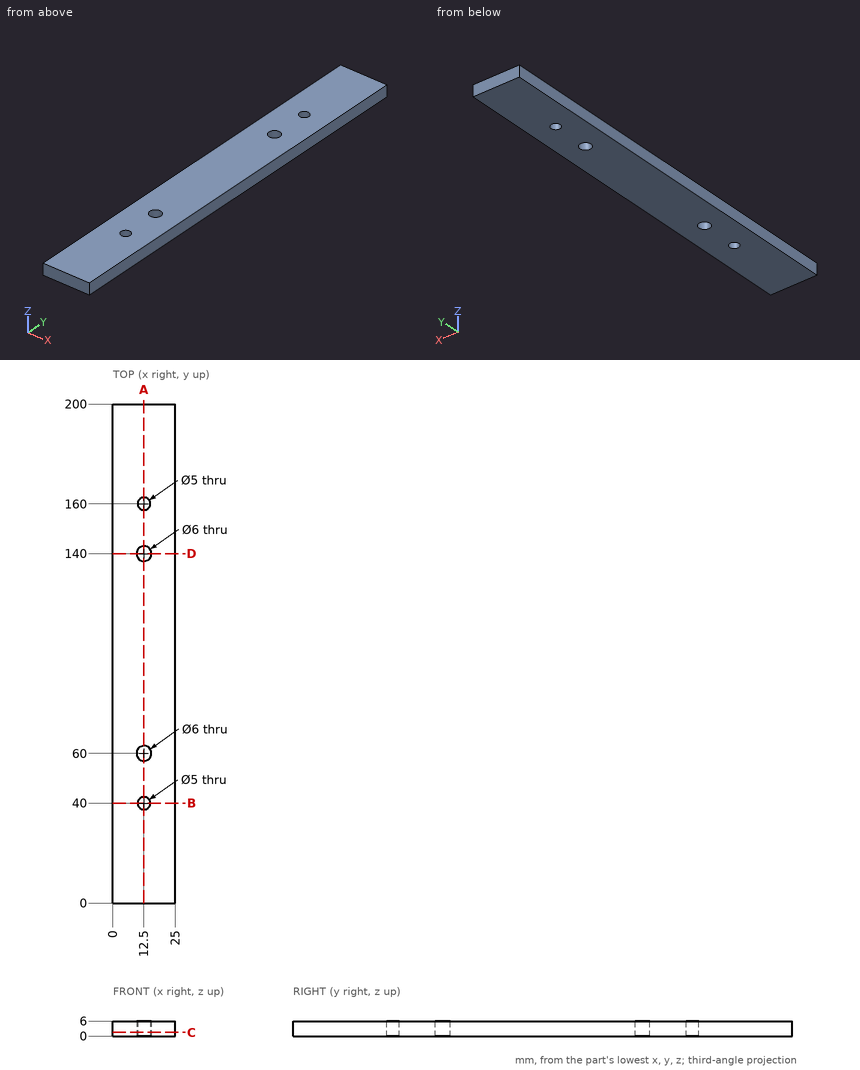
Check sheet for the drawn part. Datum: minimum x, y, z corner. Units: mm. Round coordinates to 2 decimals unless told otherwise and drop trailing zeros. Order: outer loops, then holes, each group sorted by start corner. A loop starts at its lowest first (then second) coordinate and runs counter-clockwise, first axis right, second up.
1. Section check C-C on z = 1.45. Record the cut outline in (x, y), then the cut area to 3 significant figures.
Final values:
outline: (0, 0) - (25, 0) - (25, 200) - (0, 200) - close; hole circle Ø6 at (12.5, 60); hole circle Ø6 at (12.5, 140); hole circle Ø5 at (12.5, 40); hole circle Ø5 at (12.5, 160)
area: 4,900 mm2
2. Section check A-A on x = 12.5. Record the cut outline in (y, z), then the cut area to 3 significant figures.
Final values:
outline: (0, 0) - (37.5, 0) - (37.5, 6) - (0, 6) - close; (42.5, 0) - (57, 0) - (57, 6) - (42.5, 6) - close; (63, 0) - (137, 0) - (137, 6) - (63, 6) - close; (143, 0) - (157.5, 0) - (157.5, 6) - (143, 6) - close; (162.5, 0) - (200, 0) - (200, 6) - (162.5, 6) - close
area: 1,070 mm2
3. Thickness scan on L1, parallel to Y at x = 12.5, z = 1.45; L2, parallel to Y at x = 13.5, z = 4.3; L3, parallel to X at y = 140, z = 3.55. Record the ranges inside material, lowest first.
Final values:
L1: y = 0 to 37.5, 42.5 to 57, 63 to 137, 143 to 157.5, 162.5 to 200
L2: y = 0 to 37.71, 42.29 to 57.17, 62.83 to 137.17, 142.83 to 157.71, 162.29 to 200
L3: x = 0 to 9.5, 15.5 to 25
4. Section check B-B on y = 40. Record the cut outline in (x, z).
Final values:
outline: (0, 0) - (10, 0) - (10, 6) - (0, 6) - close; (15, 0) - (25, 0) - (25, 6) - (15, 6) - close
5. Section check D-D on y = 140. Record the cut outline in (x, z), then the cut area to 3 significant figures.
Final values:
outline: (0, 0) - (9.5, 0) - (9.5, 6) - (0, 6) - close; (15.5, 0) - (25, 0) - (25, 6) - (15.5, 6) - close
area: 114 mm2
